Answer from the drawing. Dimensions are ordinates in mm from the lowest x, y and z of the part. Coordinates: 2 decimals unless noted, no trailing zeros. Order: outer loops, then holes, each group sorted by start corner. A loop starts at its lowest first (then second) coordinate and runs counter-clockwise, first axis right, second up. Notation, with made-up numbers: (73, 14.5) - (127, 14.5) arc R21 ccw to (127, 34.5) - close; hole circle Ø6 at (53.25, 2). An arc over 180 degrees is marked (long way). Use a Markdown table: item, result. Add a question column.
Item 1: The part is cut by section D-D, the plane x = 31. Give the vertices of the cut face in (y, z).
Item 2: Flat-ended cylindrical pins translate along their axes: P1, Ø0.9, axis at x = 6.5, z = 1, coming from the -Y side; P2, Ø0.9, axis at x = 7, z = 2, coming from the -Y side; P3, Ø0.9, axis at x = 6.5, z = 1, coming from the +Y side. Find the tip coordinate at first contact, or state that the pin passes through.
Item 3: The part is cut by section A-A, the plane y = 57.5. Give the vertices of the cut face in (x, z).
Item 4: Find the intervals of material crossed by line 1 along X through (y, z) = (40, 1.8); line 2 along X through (y, z) = (16.5, 2); line 3 along X through (y, z) = (21.5, 2.8), in increasing order.
Item 5: The part is cut by section B-B, the plane x = 13. Give the vertices of the cut face in (y, z).
Item 6: The part is cut by section C-C, the plane z = 0.85. State how many separate pieces and enclosed holes the cut face has, then the cut area to 3 significant figures.
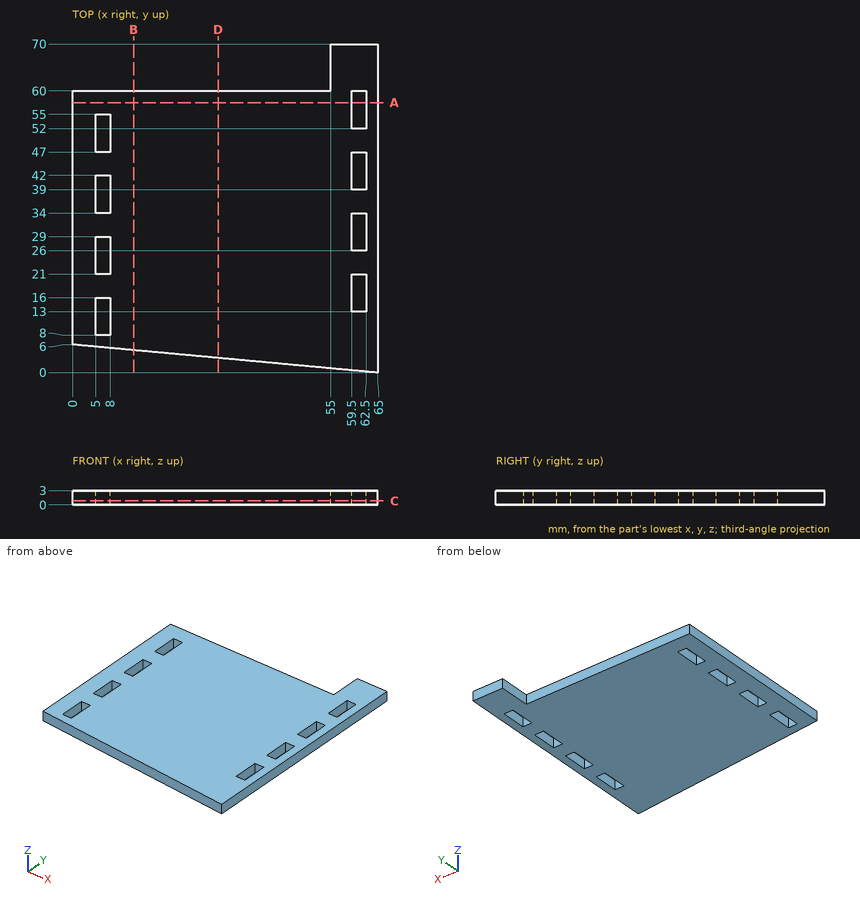
Solution:
| question | item | result |
|---|---|---|
| 1 | outline | (3.14, 0) - (60, 0) - (60, 3) - (3.14, 3) - close |
| 2 | P1 | stops at y = 5.36 |
| 2 | P2 | stops at y = 5.31 |
| 2 | P3 | stops at y = 60 |
| 3 | outline | (0, 0) - (59.5, 0) - (59.5, 3) - (0, 3) - close; (62.5, 0) - (65, 0) - (65, 3) - (62.5, 3) - close |
| 4 | line 1 | x = 0 to 5, 8 to 59.5, 62.5 to 65 |
| 4 | line 2 | x = 0 to 59.5, 62.5 to 65 |
| 4 | line 3 | x = 0 to 5, 8 to 65 |
| 5 | outline | (4.8, 0) - (60, 0) - (60, 3) - (4.8, 3) - close |
| 6 | separate pieces | 1 |
| 6 | enclosed holes | 8 |
| 6 | area | 3,610 mm2 |
